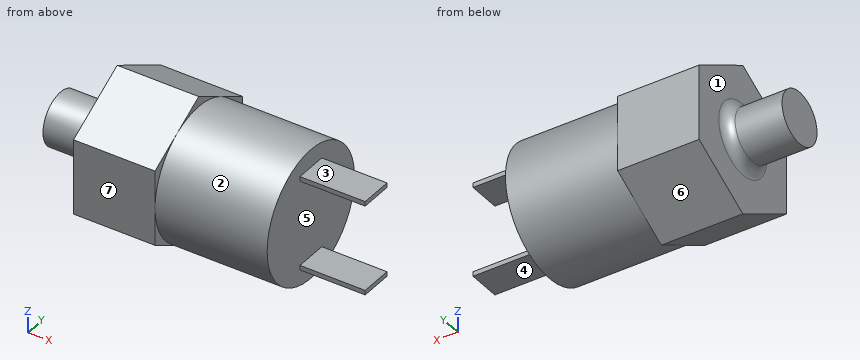
```python
from build123d import *

# Parameters (mm, degrees)
BOSS_EXTRUDE1_DEPTH = 15.875
SKETCH2_R           = 12.7
BOSS_EXTRUDE2_DEPTH = 21.844
SKETCH3_R           = 5.08
BOSS_EXTRUDE3_DEPTH = 11.049
FILLET1_R           = 1.905
SKETCH4_W           = 0.889
SKETCH4_H           = 6.35
BOSS_EXTRUDE4_DEPTH = 12.7


with BuildPart() as part:
    # Sketch1 → Boss-Extrude1 (new body)
    with BuildSketch(Plane(origin=(0, 0, 0), x_dir=(0, 0, -1), z_dir=(1, 0, 0))):
        Polygon((14.664696837, 0), (7.332348419, 12.7), (-7.332348419, 12.7), (-14.664696837, 0), (-7.332348419, -12.7), (7.332348419, -12.7), align=None)
    extrude(amount=BOSS_EXTRUDE1_DEPTH)

    # Sketch2 → Boss-Extrude2 (add)
    with BuildSketch(Plane(origin=(15.875, 0, 0), x_dir=(0, 0, -1), z_dir=(1, 0, 0))):
        with Locations(Location((0, 0, 0), (0, 0, 150))):
            Circle(SKETCH2_R)
    extrude(amount=BOSS_EXTRUDE2_DEPTH)

    # Sketch3 → Boss-Extrude3 (add)
    with BuildSketch(Plane.ZY):
        with Locations(Location((0, 0, 0), (0, 0, 180))):
            Circle(SKETCH3_R)
    extrude(amount=BOSS_EXTRUDE3_DEPTH)

    # Fillet1
    fillet1_edges = [part.edges().sort_by_distance(p)[0] for p in [
        (0, 0, 5.08),
    ]]
    fillet(fillet1_edges, radius=FILLET1_R)

    # Sketch4 → Boss-Extrude4 (add)
    with BuildSketch(Plane(origin=(37.719, 0, 0), x_dir=(0, 0, -1), z_dir=(1, 0, 0))):
        with Locations((-8.763, 0)):
            Rectangle(SKETCH4_W, SKETCH4_H)
        with Locations((8.763, 0)):
            Rectangle(SKETCH4_W, SKETCH4_H)
    extrude(amount=BOSS_EXTRUDE4_DEPTH)


solid = part.part
```
Read the model definition and answer for the solid it produces. Units are mm, in the model's axes. Face numbers are marked on the shaded views. A direction names the side the tool comes from. Give positions to 0.01 mm unless a question says otherwise; leave off trailing zeros. Write each loop counter-clockwise with the first axis right and the second up, starting at its lowest first coordinate (ties: lowest second). Pieces come first, ordered by that corner, then holes. Notation, with made-up numbers: M 76.5,65 L 89.5,65 A19 cw 89.5,72 Z; hole C 68,9 d9. An arc over 180 degrees is marked long. Put each result on its own line as item: value. Start each with the question number.
1. Which of the six approach directions +Z, -Z, +X, -X, +Y, -Y give full straight-line access (tool end or side, diameter ignored) to the marked faces 1, 2, 3 and 4?
2. The part is cut by section B-B, the plane y = 8.5. Give the vertices of the cut face in (x, z) (3 decimals), and give its area (3 significant figures).
3. The part is cut by section A-A, the plane x = 2. Give the vertices of the cut face in (y, z), and give its area (3 significant figures).
4. Each of these flat-tipped pins is pushed along its axis until it touches: pin 1 Ø3 at (y, z) = (0.5, -13.5) entering from +X; pin 2 Ø3 at (x, y) = (42, -1) entering from -Z; pin 3 Ø3 at (x, y) = (43.5, -0.5) entering from +Z. Where does it stop, or does it pass through?
5. Consider line 1 along X through (y, z) = (5, -4.75); line 2 along Z through (x, y) = (24, -11); line 3 along Y through (x, z) = (-9, 0.25). Determine where each line is inside the solid, lowest interval first.
6. For a pull along Z with two mould halves and no side action, classify the marked faces 5, 6 and 7 as released by +Z, released by -Z, zero draft, split by the parting line, or undercut.
Final values:
1. face 1: -X
1. face 2: +X
1. face 3: +Z, +X, +Y, -Y
1. face 4: -Z, +X, +Y, -Y
2. outline: M 0,-9.757 L 15.875,-9.757 L 15.875,-9.436 L 37.719,-9.436 L 37.719,9.436 L 15.875,9.436 L 15.875,9.757 L 0,9.757 Z
2. area: 722 mm²
3. outline: M -12.7,-7.33 L 0,-14.66 L 12.7,-7.33 L 12.7,7.33 L 0,14.66 L -12.7,7.33 Z
3. area: 559 mm²
4. pin 1: stops at x = 37.72
4. pin 2: stops at z = -9.21
4. pin 3: stops at z = 9.21
5. line 1: x = 0 to 37.72
5. line 2: z = -6.35 to 6.35
5. line 3: y = -5.07 to 5.07
6. face 5: undercut
6. face 6: released by -Z
6. face 7: zero draft
